from build123d import *


with BuildPart() as f1:
    # F0 (on Front) → F1 (revolve)
    with BuildSketch(Plane.XZ):
        with BuildLine():
            Line((0, 21.543375), (0, 0))
            Line((0, 0), (1.5875, 0))
            Line((1.5875, 0), (1.5875, 3.175))
            Line((1.5875, 3.175), (7.9375, 3.175))
            ThreePointArc((7.9375, 3.175), (8.73125, 3.96875), (7.9375, 4.7625))
            ThreePointArc((7.9375, 4.7625), (4.963216, 12.359188), (7.9375, 19.955875))
            ThreePointArc((7.9375, 19.955875), (8.73125, 20.749625), (7.9375, 21.543375))
            Line((7.9375, 21.543375), (0, 21.543375))
        make_face()
    revolve(axis=Axis((0, 0, 10.771688), (0, 0, -1)))


solid = f1.part
Verification items for the finished model (mm, model axes). Give positions to 0.01 mm unless a question says otherwise; leave off trailing zeros. Write each loop counter-clockwise with the first axis right and the second up, starting at its lowest first coordinate (ties: lowest second). Pieces come first, ordered by that corner, then holes. Notation, with made-up numbers: M 29.5,83 L 39.5,83 A21 ccw 39.5,88 Z; hole C -1.5,-6.75 d5. An arc over 180 degrees is marked long. Use CSV: the item, a comma, the result in double quotes.
1) Go/stop test with flat-tipped pins: pin 1 Ø1 at (x, z) = (1, 10) entering from -Y; pin 2 Ø3 at (y, z) = (4.5, 14.5) entering from -X; pin 3 Ø5 at (y, z) = (-4.5, 11.5) entering from +X. Record where each tip stops, or that it passes through.
Final values:
pin 1,"y = -5.26"
pin 2,"x = -4.29"
pin 3,"x = 4.62"
2) Release check for a two-part mould opening along Y. For faces 1 (the face through (-2, 0, 3.175)), 2 (the face through (-0.34, 1.55, 1.61)) record: released by +Y, released by -Y, zero draft, split by the parting line, or undercut.
Final values:
face 1,"zero draft"
face 2,"split by the parting line"
3) Cross-section at C-C (z = 19). Enter the section's corners in (x, y), plus the area to 3 significant figures.
Final values:
outline,"C 0,0 d14.29"
area,"160 mm²"
4) Material ranges on line 1 along Z through (x, y) = (-5.25, 6); line 2 along Z through (x, y) = (-4, -5.25) (3 decimals); line 3 along Z through (x, y) = (-1.75, -2.5) (3 decimals), recorded low to high.
Final values:
line 1,"3.18 to 4.76, 19.96 to 21.54"
line 2,"3.175 to 6.532, 18.186 to 21.543"
line 3,"3.175 to 21.543"
5) Cross-section at A-A (y = 0). Enter the section's corners in (x, z) (1 decimal).
Final values:
outline,"M -7.9,3.2 L -1.6,3.2 L -1.6,0 L 1.6,0 L 1.6,3.2 L 7.9,3.2 A0.8 ccw 7.9,4.8 A11.2 cw 7.9,20 A0.8 ccw 7.9,21.5 L -7.9,21.5 A0.8 ccw -7.9,20 A11.2 cw -7.9,4.8 A0.8 ccw Z"
6) Cross-section at D-D (z = 5.5). Enter the section's corners in (x, y).
Final values:
outline,"C 0,0 d14.62"
